Input: part model. Units: mm. Frame: model coordinates. Face numbers are marked on the shaded views. A direction names the side the tool comes from. Give positions to 0.01 mm unless a question says otherwise; leave off trailing zeros. Order: outer loops, then holes, each group sorted by start corner. A loop starts at its lowest first (then second) coordinate and runs counter-clockwise, first axis right, second up. Notation, with made-up numbers: (-0.75, -14) - (33.25, -14) arc R20 ccw to (33.25, 6) - close; hole circle Ø7 at (88, -5.75). An arc over 180 degrees is marked (long way). Use a Markdown table: item, result.
from build123d import *

# Parameters (mm, degrees)
PAD063_DEPTH         = 10
SKETCH257_R          = 2.75
POCKET173_DEPTH      = 12.001
POCKET173_DEPTH_BACK = 9.001
FILLET011_R          = 2.5


with BuildPart() as part:
    # Sketch256 → Pad063 (new body, symmetric)
    with BuildSketch(Plane.XZ):
        Polygon((-12, 8.5), (9, 8.5), (9, -65), (0, -65), (0, -58), (-2, -58), (-2, -52), (0, -52), (0, -30), (2, -28.831445), (2, -3.5), (-2, 0.5), (-12, 0.5), align=None)
    extrude(amount=PAD063_DEPTH, both=True)

    # Sketch258 → Groove007 (revolve, cut)
    with BuildSketch(Plane.XZ):
        with BuildLine():
            Line((-12, 0.5), (-12, -8.5))
            Line((-12, -8.5), (2, -8.5))
            Line((2, -3.5), (2, -8.5))
            ThreePointArc((2, -3.5), (0.828427, -0.671573), (-2, 0.5))
            Line((-12, 0.5), (-2, 0.5))
        make_face()
    revolve(axis=Axis((0, 0, 165.5), (1, 0, 0)), mode=Mode.SUBTRACT)

    # Sketch257 → Pocket173 (cut, two sides)
    with BuildSketch(Plane.YZ) as pocket173_sk:
        with Locations((0, -55)):
            Circle(SKETCH257_R)
    extrude(amount=-POCKET173_DEPTH, mode=Mode.SUBTRACT)
    extrude(pocket173_sk.sketch, amount=POCKET173_DEPTH_BACK, mode=Mode.SUBTRACT)

    # Fillet011
    fillet011_edges = [part.edges().sort_by_distance(p)[0] for p in [
        (-12, -5.002299, 0.575845),
        (-12, 5.002299, 0.575845),
        (-12, 10, 4.651655),
        (-12, -10, 4.651655),
        (-12, 0, 8.5),
        (-1.5, -10, 8.5),
        (-1.5, 10, 8.5),
        (9, 0, 8.5),
        (9, 10, -28.25),
        (9, -10, -28.25),
        (2, 0, -28.831445),
    ]]
    fillet(fillet011_edges, radius=FILLET011_R)


with BuildPart() as part_1:
    # Body022056 placement: moved
    add(part.part.moved(Location((137, 0, -82))))


solid = part_1.part
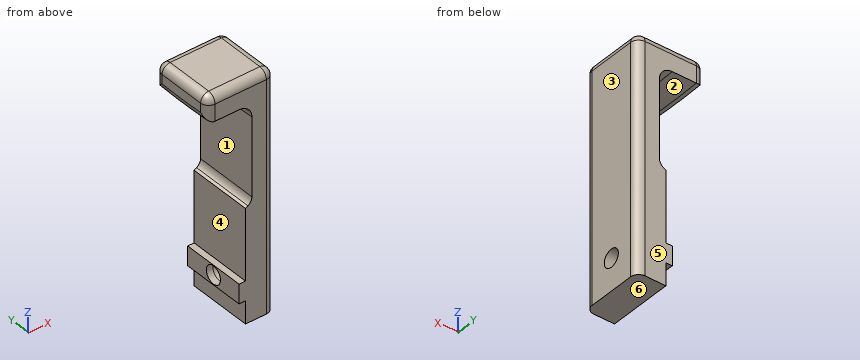
1. Section query A-A (y = 0). Return loops of the section in (x, z).
Response:
| item | result |
|---|---|
| outline | (125, -79) arc R2.5 ccw to (127.5, -81.5) - (135, -81.5) arc R4 cw to (139, -85.5) - (139, -109.4) arc R2.5 cw to (137.76, -111.56) - (137, -112) - (137, -134) - (135, -134) - (135, -134.25) - (146, -134.25) - (146, -76) arc R2.5 ccw to (143.5, -73.5) - (127.5, -73.5) arc R2.5 ccw to (125, -76) - close; (135, -140) - (137, -140) - (137, -147) - (146, -147) - (146, -139.75) - (135, -139.75) - close |
2. Mould query, pull axis Z, two halves, no side actions, for the marked faces 4, 5 and 6. Classes: pulls with the +Z half, pulls with the -Z half, needs draft (parallel to the pull), parting line crosses it, or undercut.
Response:
| item | result |
|---|---|
| face 4 | undercut |
| face 5 | needs draft |
| face 6 | pulls with the -Z half |
3. Pin query (flat end, axial travel): pin 1 (7 mm diameter, centred on y = 0, z = -137, fed in from -X); pin 2 (1.6 mm diameter, centred on x = 136, y = -4, fed in from -Z); pin 3 (5 mm diameter, centred on y = 5, z = -105.5, fed in from -X). Return the tip coordinate at first contact, or that it passes through.
Response:
| item | result |
|---|---|
| pin 1 | stops at x = 135 |
| pin 2 | stops at z = -140 |
| pin 3 | stops at x = 139 |
4. Section query B-B (x = 141.75). Return loops of the section in (y, z).
Response:
| item | result |
|---|---|
| outline | (-10, -147) - (10, -147) - (10, -76) arc R2.5 ccw to (7.5, -73.5) - (-7.5, -73.5) arc R2.5 ccw to (-10, -76) - close; hole circle Ø5.5 at (0, -137) |
5. Section query D-D (z = -98.5). Return loops of the section in (x, y).
Response:
| item | result |
|---|---|
| outline | (139, -10) - (143.5, -10) arc R2.5 ccw to (146, -7.5) - (146, 7.5) arc R2.5 ccw to (143.5, 10) - (139, 10) - close |
6. Material intervals for line 1 along Z through (x, y) = (142.75, 0); line 2 along Y through (x, z) = (135.7, -137); line 3 along Z through (x, y) = (135.6, 0), sorted ascending.
Response:
| item | result |
|---|---|
| line 1 | z = -147 to -139.75, -134.25 to -73.5 |
| line 2 | y = -10 to -2.75, 2.75 to 10 |
| line 3 | z = -140 to -139.75, -134.25 to -134, -81.55 to -73.5 |
7. Set-up query: the marked faces 1, 2 and 3. Return all of +Z, -Z, +X, -X, +Y, -Y with unobstructed straight access to the full face (end or side cutting, diameter ignored); none if empty.
Response:
| item | result |
|---|---|
| face 1 | -X, +Y, -Y |
| face 2 | -Z, -X |
| face 3 | +Z, -Z, +X, +Y, -Y |
8. Section query C-C (z = -137). Return loops of the section in (x, y), then the cut area to 3 significant figures.
Response:
| item | result |
|---|---|
| outline | (135, -10) - (143.5, -10) arc R2.5 ccw to (146, -7.5) - (146, -2.75) - (135, -2.75) - close; (135, 2.75) - (146, 2.75) - (146, 7.5) arc R2.5 ccw to (143.5, 10) - (135, 10) - close |
| area | 157 mm^2 |
